Geometry: see drawing. Coordinates: mm, zero at the bounding-box minimum. Round coordinates to 2 decimals unless told otherwise and drop trailing zeros. Order: outer loops, then holes, each group sorted by start corner. A loop starts at its lowest first (then second) coordinate and runs counter-clockwise, first axis right, second up. Notation, with made-up numbers: (80.25, 54.25) -> (94.25, 54.25) arc R29 ccw to (94.25, 75.25) -> close; hole circle Ø7 at (8, -2). An arc over 180 degrees is marked (long way). Use a Markdown table: item, result.
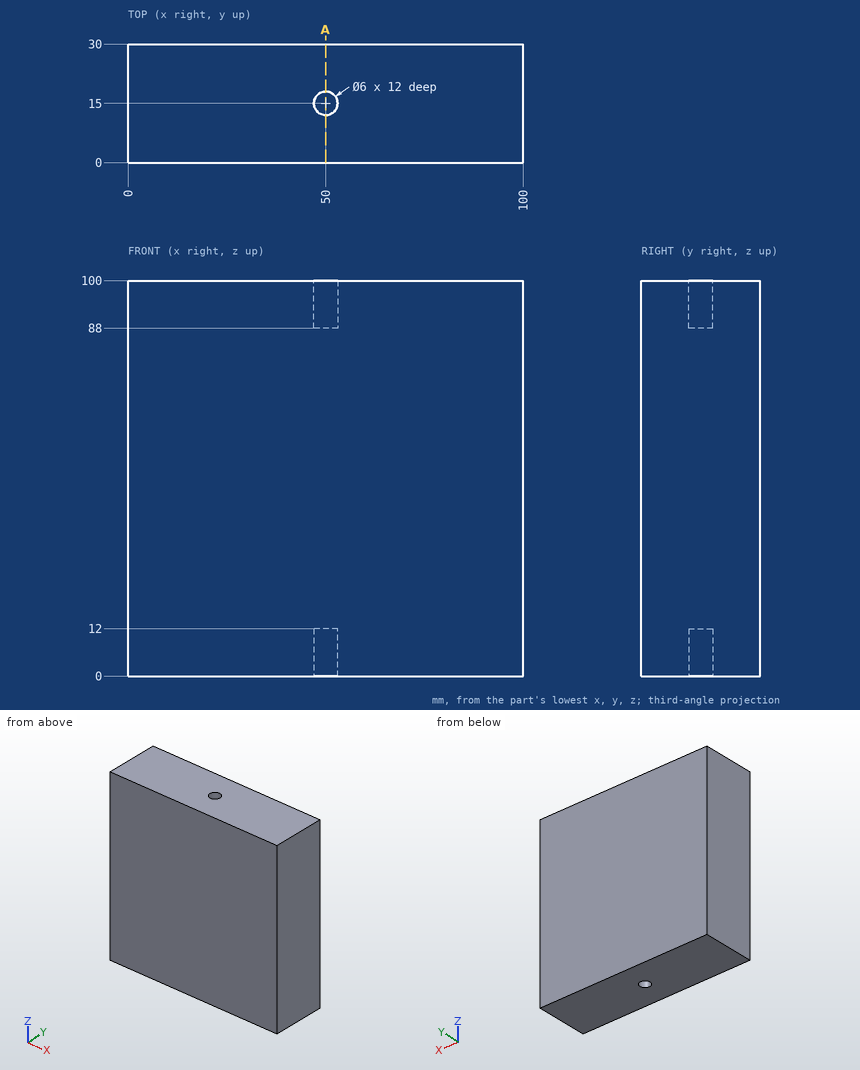
1) Ray query, probe 1 along Y at (x, z) = (50, 93); probe 2 along X at (y, z) = (15, 6.75). Return the intervals inside material, ascending.
Answer key:
| item | result |
|---|---|
| probe 1 | y = 0 to 12, 18 to 30 |
| probe 2 | x = 0 to 47, 53 to 100 |
2) Contact query for flat-ended pins moving along their axis: P1, Ø12, axis at x = 70.5, y = 10.5, coming from the -Z side; P2, Ø5.5, axis at x = 50, y = 15, coming from the -Z side. Output: stop coordinate, or through.
Answer key:
| item | result |
|---|---|
| P1 | stops at z = 0 |
| P2 | stops at z = 12 |
3) Cut plane A-A on x = 50. Return loops of the section in (y, z), and give its area (3 significant figures).
Answer key:
| item | result |
|---|---|
| outline | (0, 0) -> (12, 0) -> (12, 12) -> (18, 12) -> (18, 0) -> (30, 0) -> (30, 100) -> (18, 100) -> (18, 88) -> (12, 88) -> (12, 100) -> (0, 100) -> close |
| area | 2,860 mm^2 |
